Autodesk Inventor part; units mm, degrees
ref_plane "YZ Plane" through (0, 0, 0) normal (1, 0, 0) x (0, 1, 0)
ref_plane "XZ Plane" through (0, 0, 0) normal (0, 1, 0) x (-1, 0, 0)
ref_plane "XY Plane" through (0, 0, 0) normal (0, 0, 1) x (1, 0, 0)
sketch "Sketch1" plane through (0, 0, 0) normal (0, 0, 1) x (1, 0, 0)
  circle A0 centre (0, 0) radius 4
  dimension "Diameter" = 8
extrude "Extrusion1" add sketch "Sketch1" along normal blind 65.04
sketch "Sketch2" plane through (0, 0, 65.04) normal (0, 0, 1) x (1, 0, 0)
  circle A0 centre (0, 0) radius 4
extrude "Extrusion2" add sketch "Sketch2" along normal blind 4.96 draft 45
sketch "Sketch3" plane through (0, 0, 70) normal (0, 0, 1) x (1, 0, 0)
  circle A0 centre (0, 0) radius 8.96
  circle A1 centre (0, 0) radius 2.8868 construction
  line L0 (1.2084, 2.6217) -> (2.8746, 0.2644)
  line L1 (2.8746, 0.2644) -> (1.6662, -2.3573)
  line L2 (1.6662, -2.3573) -> (-1.2084, -2.6217)
  line L3 (-1.2084, -2.6217) -> (-2.8746, -0.2644)
  line L4 (-2.8746, -0.2644) -> (-1.6662, 2.3573)
  line L5 (-1.6662, 2.3573) -> (1.2084, 2.6217)
  dimension "Hex_Width" = 5
extrude "Extrusion3" cut sketch "Sketch3" against normal blind 3 contours L0 L1 L2 L3 L4 L5
thread "Thread1"
chamfer "Chamfer2" distance 0.8 angle 45 1 edges at (-4, 0, 0)
fillet "Fillet1" radius 0.1 1 edges at (-8.96, 0, 70)
equation "\"d10\" = Thread_Length"
equation "\"d13\" = Chamfer"
equation "\"Thread_Length\" = 45"
properties part number "SCREW,FLAT HD,P,5,M8X1"
Can you work these out from the model? Positions are in its coordinate system, mm. A direction names the side the tool comes from. Coordinates: 2 decimals unless noted, no trailing zeros. Write each loop counter-clockwise with the first axis right and the second up, starting at its lowest first coordinate (ties: lowest second). Pieces come first, ordered by that corner, then holes. Notation, with made-up numbers: (57, 59) -> (103, 59) arc R21 ccw to (103, 96) -> close; hole circle Ø1 at (-11.75, -28). An arc over 180 degrees is marked (long way). Write each question's results on one line, items separated by ' | '. Start each with the question number.
Item 1: If we section it at B-B, the plane z = 46.5: Write out the boundary of the cut face in (x, y), and give its area (3 significant figures).
Item 2: If we section it at A-A, the plane x = 0: Write out the boundary of the cut face in (y, z), and give its area (3 significant figures).
Item 3: Thinking about a two-plate mould opening in X: for faces 1 (the flat face through (0.249, -2.488, 68.521)), 2 (the flat face through (0, 0, 0)), 3 (the cylindrical face through (-0.867, 3.905, 32.47)), 4 (the flat face through (0, 0, 67)), which applies, released by +X, released by -X, zero draft, split by the parting line, or undercut?
Item 4: I'm going to push flat-ended pins straight in: P1, Ø4, axis at y = 0, z = 35, coming from the -X side; P2, Ø5, axis at x = 4, z = 21.5, coming from the +Y side; P3, Ø5, axis at x = -5.5, z = 33, coming from the +Y side; P4, Ø4, axis at x = 2, y = 1, coming from the -Z side. Where does each tip first touch, or does it pass through?
Item 5: On a 3-axis mill with a long thin cutter (end or side, diameter ignored), from which of +Z, -Z, +X, -X, +Y, -Y can I reach the whole of each face in a straight line? I mean faces 5 (the conical face through (-0.93, -4.2, 65.34)), 6 (the flat face through (-0.249, 2.488, 68.521)). Say none if no direction works.
Item 6: Please list where these lines run through material, in increasing order: probe 1 along Z at (x, y) = (-0.5, 0); probe 2 along Z at (x, y) = (1.5, 7.5); probe 3 along X at (y, z) = (-3, 43).
Answer block:
1) outline: circle Ø8 at (0, 0) | area: 50.3 mm²
2) outline: (-8.79, 69.83) -> (-4, 65.04) -> (-4, 0.8) -> (-3.2, 0) -> (3.2, 0) -> (4, 0.8) -> (4, 65.04) -> (8.79, 69.83) arc R0.1 ccw to (8.72, 70) -> (2.51, 70) -> (2.51, 67) -> (-2.51, 67) -> (-2.51, 70) -> (-8.72, 70) arc R0.1 ccw to start | area: 569 mm²
3) face 1: undercut | face 2: zero draft | face 3: split by the parting line | face 4: undercut
4) P1: x = -4 | P2: y = 3.71 | P3: y = 2.65 | P4: z = 0
5) face 5: -Z | face 6: +Z
6) probe 1: 0 to 67 | probe 2: 68.69 to 70 | probe 3: -2.65 to 2.65
